from build123d import *

# Parameters (mm, degrees)
BOSS_EXTRU_3_DEPTH            = 20
ENL_V_MAT_EXTRU_11_DEPTH      = 295.374154069
ENL_V_MAT_EXTRU_11_DEPTH_BACK = 249
ENL_V_MAT_EXTRU_12_DEPTH      = 295.374154069
ENL_V_MAT_EXTRU_12_DEPTH_BACK = 249
ENL_V_MAT_EXTRU_13_DEPTH      = 372.52143865
ENL_V_MAT_EXTRU_13_DEPTH_BACK = 249
ENL_V_MAT_EXTRU_14_DEPTH      = 372.52143865
ENL_V_MAT_EXTRU_14_DEPTH_BACK = 249
ENL_V_MAT_EXTRU_15_DEPTH      = 295.374154069
ENL_V_MAT_EXTRU_15_DEPTH_BACK = 249
ENL_V_MAT_EXTRU_16_DEPTH      = 295.374154069
ENL_V_MAT_EXTRU_16_DEPTH_BACK = 249
ENL_V_MAT_EXTRU_17_DEPTH      = 372.52143865
ENL_V_MAT_EXTRU_17_DEPTH_BACK = 249
ENL_V_MAT_EXTRU_18_DEPTH      = 372.52143865
ENL_V_MAT_EXTRU_18_DEPTH_BACK = 249


with BuildPart() as part:
    # Esquisse1 → Boss.-Extru.3 (new body)
    with BuildSketch(Plane.XY):
        Polygon((-263.060356118, 145.358531169), (-14.060356118, 145.358531169), (-14.060356118, 139.158531169), (-7.860356118, 139.158531169), (-7.860356118, -109.841468831), (-14.060356118, -109.841468831), (-14.060356118, -116.041468831), (-263.060356118, -116.041468831), (-263.060356118, -109.841468831), (-269.260356118, -109.841468831), (-269.260356118, 139.158531169), (-263.060356118, 139.158531169), align=None)
    extrude(amount=BOSS_EXTRU_3_DEPTH)

    # Esquisse4 → Enl_v. mat.-Extru.11 (cut, two sides: drawn at the far end of the back side and taken through both)
    with BuildSketch(Plane(origin=(-14.060356118, 0, 0), x_dir=(0, 0, -1), z_dir=(1, 0, 0)).offset(-ENL_V_MAT_EXTRU_11_DEPTH_BACK)):
        Polygon((-553.411816833, 139.158531169), (-20, 139.158531169), (-12.45, 139.158531169), (-12.45, 140.708531169), (-16.15, 140.708531169), (-16.15, 141.708531169), (-12.65, 145.358531169), (356.535030531, 530.365777294), (-64.826371106, 1510.451097334), (-974.77321847, 1119.243851209), align=None)
    extrude(amount=ENL_V_MAT_EXTRU_11_DEPTH + ENL_V_MAT_EXTRU_11_DEPTH_BACK, mode=Mode.SUBTRACT)

    # Esquisse8 → Enl_v. mat.-Extru.12 (cut, two sides: drawn at the far end of the back side and taken through both)
    with BuildSketch(Plane(origin=(-14.060356118, 0, 0), x_dir=(0, 0, -1), z_dir=(1, 0, 0)).offset(-ENL_V_MAT_EXTRU_12_DEPTH_BACK)):
        Polygon((533.411816833, 139.158531169), (0, 139.158531169), (-7.55, 139.158531169), (-7.55, 140.708531169), (-3.85, 140.708531169), (-3.85, 141.708531169), (-7.35, 145.358531169), (-376.535030531, 530.365777294), (44.826371106, 1510.451097334), (954.77321847, 1119.243851209), align=None)
    extrude(amount=ENL_V_MAT_EXTRU_12_DEPTH + ENL_V_MAT_EXTRU_12_DEPTH_BACK, mode=Mode.SUBTRACT)

    # Esquisse10 → Enl_v. mat.-Extru.13 (cut, two sides: drawn at the far end of the back side and taken through both)
    with BuildSketch(Plane(origin=(0, 139.158531169, 0), x_dir=(1, 0, 0), z_dir=(0, 1, 0)).offset(-ENL_V_MAT_EXTRU_13_DEPTH_BACK)):
        Polygon((-263.060356118, -20), (-263.060356118, -12.45), (-264.610356118, -12.45), (-264.610356118, -16.15), (-265.610356118, -16.15), (-269.260356118, -12.65), (-269.260356118, -20), align=None)
    extrude(amount=ENL_V_MAT_EXTRU_13_DEPTH + ENL_V_MAT_EXTRU_13_DEPTH_BACK, mode=Mode.SUBTRACT)

    # Esquisse11 → Enl_v. mat.-Extru.14 (cut, two sides: drawn at the far end of the back side and taken through both)
    with BuildSketch(Plane(origin=(0, 139.158531169, 0), x_dir=(1, 0, 0), z_dir=(0, 1, 0)).offset(-ENL_V_MAT_EXTRU_14_DEPTH_BACK)):
        Polygon((-643.553156031, -387.393505759), (-269.260356118, -7.35), (-265.813317082, -3.85), (-264.610356118, -3.85), (-264.610356118, -7.55), (-263.060356118, -7.55), (-263.060356118, 0), (-263.060356118, 533.411816833), (-1249.023765439, 940.82907325), (-1629.516565352, 20.023750658), align=None)
    extrude(amount=ENL_V_MAT_EXTRU_14_DEPTH + ENL_V_MAT_EXTRU_14_DEPTH_BACK, mode=Mode.SUBTRACT)

    # Esquisse12 → Enl_v. mat.-Extru.15 (cut, two sides: drawn at the far end of the back side and taken through both)
    with BuildSketch(Plane.ZY.offset(263.060356118).offset(-ENL_V_MAT_EXTRU_15_DEPTH_BACK)):
        Polygon((20, -109.841468831), (12.45, -109.841468831), (12.45, -111.391468831), (16.15, -111.391468831), (16.15, -112.391468831), (12.65, -116.041468831), (20, -116.041468831), align=None)
    extrude(amount=ENL_V_MAT_EXTRU_15_DEPTH + ENL_V_MAT_EXTRU_15_DEPTH_BACK, mode=Mode.SUBTRACT)

    # Esquisse13 → Enl_v. mat.-Extru.16 (cut, two sides: drawn at the far end of the back side and taken through both)
    with BuildSketch(Plane.ZY.offset(263.060356118).offset(-ENL_V_MAT_EXTRU_16_DEPTH_BACK)):
        Polygon((376.535030531, -501.048714956), (7.35, -116.041468831), (3.85, -112.391468831), (3.85, -111.391468831), (7.55, -111.391468831), (7.55, -109.841468831), (0, -109.841468831), (-533.411816833, -109.841468831), (-954.77321847, -1089.92678887), (-44.826371106, -1481.134034995), align=None)
    extrude(amount=ENL_V_MAT_EXTRU_16_DEPTH + ENL_V_MAT_EXTRU_16_DEPTH_BACK, mode=Mode.SUBTRACT)

    # Esquisse15 → Enl_v. mat.-Extru.17 (cut, two sides: drawn at the far end of the back side and taken through both)
    with BuildSketch(Plane(origin=(0, 139.158531169, 0), x_dir=(1, 0, 0), z_dir=(0, 1, 0)).offset(-ENL_V_MAT_EXTRU_17_DEPTH_BACK)):
        Polygon((-14.060356118, 0), (-14.060356118, -7.55), (-12.510356118, -7.55), (-12.510356118, -3.85), (-11.510356118, -3.85), (-7.860356118, -7.35), (-7.860356118, 0), align=None)
    extrude(amount=ENL_V_MAT_EXTRU_17_DEPTH + ENL_V_MAT_EXTRU_17_DEPTH_BACK, mode=Mode.SUBTRACT)

    # Esquisse16 → Enl_v. mat.-Extru.18 (cut, two sides: drawn at the far end of the back side and taken through both)
    with BuildSketch(Plane(origin=(0, 139.158531169, 0), x_dir=(1, 0, 0), z_dir=(0, 1, 0)).offset(-ENL_V_MAT_EXTRU_18_DEPTH_BACK)):
        Polygon((377.146890007, 356.535030531), (-7.860356118, -12.65), (-11.510356118, -16.15), (-12.510356118, -16.15), (-12.510356118, -12.45), (-14.060356118, -12.45), (-14.060356118, -20), (-14.060356118, -553.411816833), (966.024963922, -974.77321847), (1357.232210047, -64.826371106), align=None)
    extrude(amount=ENL_V_MAT_EXTRU_18_DEPTH + ENL_V_MAT_EXTRU_18_DEPTH_BACK, mode=Mode.SUBTRACT)


solid = part.part
Model file for the job. Use its own axes, mm. A direction names the side the tool comes from. Coordinates: 2 decimals unless noted, no trailing zeros. Order: outer loops, then holes, each group sorted by start corner. A loop starts at its lowest first (then second) coordinate and runs counter-clockwise, first axis right, second up. Notation, with made-up numbers: M 85,-27.5 L 91,-27.5 A21 ccw 91,-8.5 Z; hole C 82,-29 d2. An arc over 180 degrees is marked long. Return JSON: item names as keys, results as strings.
1. Saw through at A-A (x = -54). Give the cut face in (y, z).
Ans:
{"outline": "M -116.04,7.35 L -112.39,3.85 L -111.39,3.85 L -111.39,7.55 L -109.84,7.55 L -109.84,0 L 139.16,0 L 139.16,7.55 L 140.71,7.55 L 140.71,3.85 L 141.71,3.85 L 145.36,7.35 L 145.36,12.65 L 141.71,16.15 L 140.71,16.15 L 140.71,12.45 L 139.16,12.45 L 139.16,20 L -109.84,20 L -109.84,12.45 L -111.39,12.45 L -111.39,16.15 L -112.39,16.15 L -116.04,12.65 Z"}
2. Drill centre lines: probe 1 along Y at (x, z) = (-199, 12.5); probe 2 along Y at (x, z) = (-253.5, 16); probe 3 along X at (y, z) = (73, 15). Where is each one in solid material? Low to high.
Ans:
{"probe 1": "-116.04 to -111.39, -109.84 to 139.16, 140.71 to 145.36", "probe 2": "-112.55 to -111.39, -109.84 to 139.16, 140.71 to 141.86", "probe 3": "-266.81 to -264.61, -263.06 to -14.06, -12.51 to -10.31"}
3. Saw through at B-B (y = -90). Give the cut face in (x, z).
Ans:
{"outline": "M -269.26,7.35 L -265.81,3.85 L -264.61,3.85 L -264.61,7.55 L -263.06,7.55 L -263.06,0 L -14.06,0 L -14.06,7.55 L -12.51,7.55 L -12.51,3.85 L -11.51,3.85 L -7.86,7.35 L -7.86,12.65 L -11.51,16.15 L -12.51,16.15 L -12.51,12.45 L -14.06,12.45 L -14.06,20 L -263.06,20 L -263.06,12.45 L -264.61,12.45 L -264.61,16.15 L -265.61,16.15 L -269.26,12.65 Z"}
4. Pull direction Y, two halves, no side cores. Call faces 1 (the face through (-140, 139.159, 16)), 2 (the face through (-263.06, 13, 16)), 3 (the face through (-266, -109.841, 10)): +Y half, -Y half, draft (parallel to the pull), parting line (faces both ways), or undercut.
Ans:
{"face 1": "undercut", "face 2": "draft", "face 3": "-Y half"}
5. Tool access for faces 4 (the face through (-11, -109.841, 10)), 5 (the face through (-14.06, 13, 4)), 6 (the face through (-263.06, -113, 10)), 7 (the face through (-140, 139.159, 4)): list every direction of +Z, -Z, +X, -X, +Y, -Y with a clear straight run to the whole face (end or side of a thin tool).
Ans:
{"face 4": "+Z, -Z, +X, -Y", "face 5": "-Z, +Y, -Y", "face 6": "+Z, -Z, -X, -Y", "face 7": "-Z, +X, -X"}
6. Flat gauge pins, fed straight in: pin 1 (1.5 mm diameter, centred on x = -220.5, z = 15, fed in from -Y); pin 2 (2 mm diameter, centred on y = 12.5, z = 2.5, fed in from +X); pin 3 (4 mm diameter, centred on x = -170, z = 4, fed in from +Y). Where does each tip first touch, or does it go through?
Ans:
{"pin 1": "y = -114.37", "pin 2": "x = -14.06", "pin 3": "y = 143.95"}
